The model under review builds one solid part; all positions refer to its coordinate system, in mm. A direction names the side the tool comes from. Round coordinates to 2 decimals unless told otherwise and drop trailing zeros. Loops run counter-clockwise (first coordinate to the right, second up) from the corner with the lowest first, then second, coordinate; pieces in that order, holes last. Notation, with made-up numbers: M -40,55 L -24,55 A25 cw -24,73 Z; hole C 25,69 d8. An arc over 180 degrees is marked long. Use a Markdown table: item, result. Add a question column.
```python
from build123d import *

# Parameters (mm, degrees)
SKETCH_1_R          = 5
EXTRUDE_1_DEPTH     = 5
SKETCH_2_R          = 2.5
EXTRUDE_2_DEPTH     = 1
SKETCH_3_R          = 5
EXTRUDE_3_DEPTH     = 5
SKETCH_4_R          = 2
CUT_EXTRUDE_1_DEPTH = 16


with BuildPart() as part:
    # Эскиз1 → Бобышка-Вытянуть1 (new body)
    with BuildSketch(Plane(origin=(0, 0, 0), x_dir=(0, 0, -1), z_dir=(1, 0, 0))):
        Circle(SKETCH_1_R)
    extrude(amount=EXTRUDE_1_DEPTH)

    # Эскиз2 → Бобышка-Вытянуть2 (add)
    with BuildSketch(Plane(origin=(5, 0, 0), x_dir=(0, 0, -1), z_dir=(1, 0, 0))):
        Circle(SKETCH_2_R)
    extrude(amount=EXTRUDE_2_DEPTH)

    # Эскиз3 → Бобышка-Вытянуть3 (add)
    with BuildSketch(Plane(origin=(6, 0, 0), x_dir=(0, 0, -1), z_dir=(1, 0, 0))):
        Circle(SKETCH_3_R)
    extrude(amount=EXTRUDE_3_DEPTH)

    # Эскиз4 → Вырез-Вытянуть1 (cut)
    with BuildSketch(Plane(origin=(11, 0, 0), x_dir=(0, 0, -1), z_dir=(1, 0, 0))):
        Circle(SKETCH_4_R)
    extrude(amount=-CUT_EXTRUDE_1_DEPTH, mode=Mode.SUBTRACT)


solid = part.part
```
(1) Draft analysis for pull direction Z (two halves, no side actions). For faces 1 (the face through (6, -2, 0)), 2 (the face through (5, -2, -2)), 3 (the face through (2.46, -4.88, 1.08)), state which applies: released by +Z, released by -Z, zero draft, split by the parting line, or undercut.
(2) Consider section D-D, the plane z = 4.25. Give the boundary of the cut face in (x, y), then the cut area to 3 significant figures.
(3) Consider section A-A, the plane y = 0. Give the boundary of the cut face in (x, z).
(4) Insertion check: pin 1 Ø1 at (y, z) = (1, -1) entering from +X; pin 2 Ø1.5 at (x, y) = (8, -1) entering from -Z; pin 3 Ø3 at (x, y) = (9.5, 2.5) entering from -Z; pin 4 Ø2 at (x, y) = (1, -2.5) entering from -Z. Each pin has a flat end and moves straight along its axis. Give the tip position at first contact, or say it passes through.
(5) For faces 4 (the face through (6, -2, -2)), 5 (the face through (11, -2.2, 0.1)), list the 3-axis set-ups (+Z, -Z, +X, -X, +Y, -Y) from which the entire face can be reached by the end or side of a thin tool; tool diameter is ignored.
(6) Consider section C-C, the plane x = 4.5. Give the boundary of the cut face in (y, z).
(7) To check wall thickness, follow probe 1 along X at (y, z) = (4.5, 0.75); probe 2 along Y at (x, z) = (7, 0); probe 3 along Y at (x, z) = (5.25, 0). State the ranges of each line that lie inside material, in increasing order.
Found:
| question | item | result |
|---|---|---|
| 1 | face 1 | undercut |
| 1 | face 2 | zero draft |
| 1 | face 3 | split by the parting line |
| 2 | outline | M 0,-2.63 L 5,-2.63 L 5,2.63 L 0,2.63 Z; M 6,-2.63 L 11,-2.63 L 11,2.63 L 6,2.63 Z |
| 2 | area | 52.7 mm^2 |
| 3 | outline | M 0,-5 L 5,-5 L 5,-2.5 L 6,-2.5 L 6,-5 L 11,-5 L 11,-2 L 0,-2 Z; M 0,2 L 11,2 L 11,5 L 6,5 L 6,2.5 L 5,2.5 L 5,5 L 0,5 Z |
| 4 | pin 1 | passes through |
| 4 | pin 2 | stops at z = -4.99 |
| 4 | pin 3 | stops at z = -4.9 |
| 4 | pin 4 | stops at z = -4.77 |
| 5 | face 4 | none |
| 5 | face 5 | +Z, -Z, +X, +Y, -Y |
| 6 | outline | C 0,0 d10; hole C 0,0 d4 |
| 7 | probe 1 | x = 0 to 5, 6 to 11 |
| 7 | probe 2 | y = -5 to -2, 2 to 5 |
| 7 | probe 3 | y = -2.5 to -2, 2 to 2.5 |
